For this review, use the dimensioned drawing (mm, ordinates from the lowest corner) and the shaded views. Coordinates: 2 decimals unless noted, no trailing zeros. Order: outer loops, then holes, each group sorted by start corner. A loop starts at its lowest first (then second) coordinate and runs counter-clockwise, first axis right, second up. Notation, with made-up numbers: M 78.5,-14.75 L 127.5,-14.75 A23 ccw 127.5,5.25 Z; hole C 48.25,45.25 d1. An arc over 180 degrees is marked long. Answer in a Markdown table with one row per item.
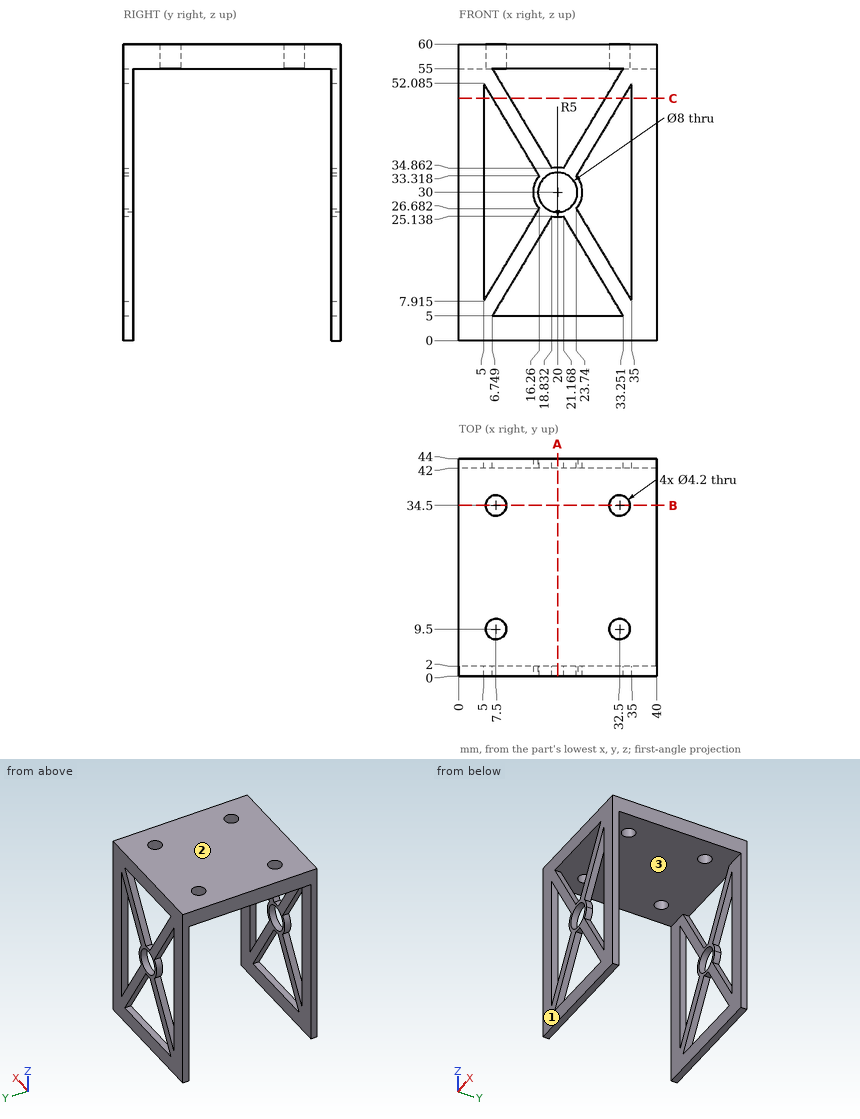
(1) Take a section at C-C (z = 49). State how many separate pieces and enclosed holes the cut face has.
Report:
| item | result |
|---|---|
| separate pieces | 8 |
| enclosed holes | 0 |
(2) The part is to be moulded in two halves that separate along Y. For the marked faces 1, 2 and 3, say which applies: +Y half, -Y half, draft (parallel to the pull), parting line (faces both ways), or undercut.
Report:
| item | result |
|---|---|
| face 1 | -Y half |
| face 2 | draft |
| face 3 | undercut |
(3) Take a section at A-A (x = 20). Write out the cut boundary in (y, z).
Report:
| item | result |
|---|---|
| outline | M 0,0 L 2,0 L 2,5 L 0,5 Z; M 0,25 L 2,25 L 2,26 L 0,26 Z; M 0,34 L 2,34 L 2,35 L 0,35 Z; M 0,55 L 44,55 L 44,60 L 0,60 Z; M 42,0 L 44,0 L 44,5 L 42,5 Z; M 42,25 L 44,25 L 44,26 L 42,26 Z; M 42,34 L 44,34 L 44,35 L 42,35 Z |
(4) Take a section at B-B (y = 34.5). Write out the cut boundary in (x, z).
Report:
| item | result |
|---|---|
| outline | M 0,55 L 5.4,55 L 5.4,60 L 0,60 Z; M 9.6,55 L 30.4,55 L 30.4,60 L 9.6,60 Z; M 34.6,55 L 40,55 L 40,60 L 34.6,60 Z |
(5) To check wall thickness, follow line 1 (Y direction, x = 32.5, z = 57.25); line 2 (X direction, y = 43.45, z = 30); line 3 (Y direction, x = 9.5, z = 11.5). State the ranges of each line that lie inside material, in increasing order. Write a range as [from, to].
Report:
| item | result |
|---|---|
| line 1 | [0, 7.4], [11.6, 32.4], [36.6, 44] |
| line 2 | [0, 5], [15, 16], [24, 25], [35, 40] |
| line 3 | [0, 2], [42, 44] |
(6) Insertion check: P1, Ø12, axis at x = 32.5, z = 27.5, coming from the +Y side; P2, Ø12, axis at x = 5, y = 32, coming from the -Z side. Each pin has a flat end and moves straight along its axis. Give the tip position at first contact, or say it passes through.
Report:
| item | result |
|---|---|
| P1 | y = 44 |
| P2 | z = 55 |
